Here's how the part is built. I have some questions about the finished solid (model axes, mm). Give positions to 0.01 mm unless a question says otherwise; leave off trailing zeros. Order: outer loops, then holes, each group sorted by start corner. A loop starts at its lowest first (then second) coordinate and runs counter-clockwise, first axis right, second up.
from build123d import *

# Parameters (mm, degrees)
SKETCH1_R           = 19.5
SKETCH1_R_2         = 15.6
BOSS_EXTRUDE1_DEPTH = 4
SKETCH3_R           = 2.65
BOSS_EXTRUDE2_DEPTH = 4


with BuildPart() as part:
    # Sketch1 → Boss-Extrude1 (new body)
    with BuildSketch(Plane.XY):
        Circle(SKETCH1_R)
        Circle(SKETCH1_R_2, mode=Mode.SUBTRACT)
    extrude(amount=BOSS_EXTRUDE1_DEPTH)

    # Sketch3 → Boss-Extrude2 (add)
    with BuildSketch(Plane.XY):
        with BuildLine():
            Line((-15.370426149, 12), (-4.335248401, 26.134615385))
            ThreePointArc((-4.335248401, 26.134615385), (0, 28.25), (4.335248401, 26.134615385))
            Line((4.335248401, 26.134615385), (15.370426149, 12))
            ThreePointArc((15.370426149, 12), (0, 19.5), (-15.370426149, 12))
        make_face()
        with Locations((0, 22.5)):
            Circle(SKETCH3_R, mode=Mode.SUBTRACT)
    extrude(amount=BOSS_EXTRUDE2_DEPTH)


solid = part.part
Q1. If we section it at A-A on y = 0: List the corners of the cut face in (x, z) for me, plus the area to 3 significant figures.
Filled sheet:
outline: (-19.5, 0) - (-15.6, 0) - (-15.6, 4) - (-19.5, 4) - close; (15.6, 0) - (19.5, 0) - (19.5, 4) - (15.6, 4) - close
area: 31.2 mm2
Q2. If we section it at C-C on z = 0.5: List the corners of the cut face in (x, y) for me.
Filled sheet:
outline: (-15.37, 12) arc R19.5 ccw (long way) to (15.37, 12) - (4.34, 26.13) arc R5.5 ccw to (-4.34, 26.13) - close; hole circle Ø31.2 at (0, 0); hole circle Ø5.3 at (0, 22.5)
Q3. If we section it at B-B on x = 0: List the corners of the cut face in (y, z) for me, plus the area to 3 significant figures.
Filled sheet:
outline: (-19.5, 0) - (-15.6, 0) - (-15.6, 4) - (-19.5, 4) - close; (15.6, 0) - (19.85, 0) - (19.85, 4) - (15.6, 4) - close; (25.15, 0) - (28.25, 0) - (28.25, 4) - (25.15, 4) - close
area: 45.0 mm2
Q4. Thinking about a two-plate mould opening in X: for faces 1 (the face through (-0.07, 28.25, 1.97)), 2 (the face through (-0.57, 19.91, 1.97)), 3 (the face through (-6, 15, 0)), 4 (the face through (9.776, 19.166, 1.972)), which applies, released by +X, released by -X, zero draft, split by the parting line, or undercut?
Filled sheet:
face 1: split by the parting line
face 2: undercut
face 3: zero draft
face 4: released by +X
Q5. I need wall thicknesses on L1, parallel to Y at x = 0, z = 3.05; L2, parallel to Y at x = 1, z = 1.65; L3, parallel to Y at x = -10, z = 1.3. Which ranges of each line are inside material? Lowest first, please.
Filled sheet:
L1: y = -19.5 to -15.6, 15.6 to 19.85, 25.15 to 28.25
L2: y = -19.47 to -15.57, 15.57 to 20.05, 24.95 to 28.16
L3: y = -16.74 to -11.97, 11.97 to 18.88
Q6. If we section it at D-D on x = -9.5: List the corners of the cut face in (y, z) for me.
Filled sheet:
outline: (-17.03, 0) - (-12.37, 0) - (-12.37, 4) - (-17.03, 4) - close; (12.37, 0) - (19.52, 0) - (19.52, 4) - (12.37, 4) - close
Q7. I'm going to push a flat-ended pin straight in: P1, Ø1.5, axis at x = 1, z = 3, coming from the -Y side. Where does the tip first touch, or does it pass through?
Filled sheet:
P1: stops at y = -19.5
